Print and shaded views of the part. All mm, measured from the part's lowest x, y and z. A direction names the side the tool comes from. Give positions to 0.01 mm unless a question says otherwise; leave off trailing zeros. Write each loop counter-clockwise with the first axis right and the second up, starting at its lowest first coordinate (ties: lowest second). Pieces come first, ordered by that corner, then holes.
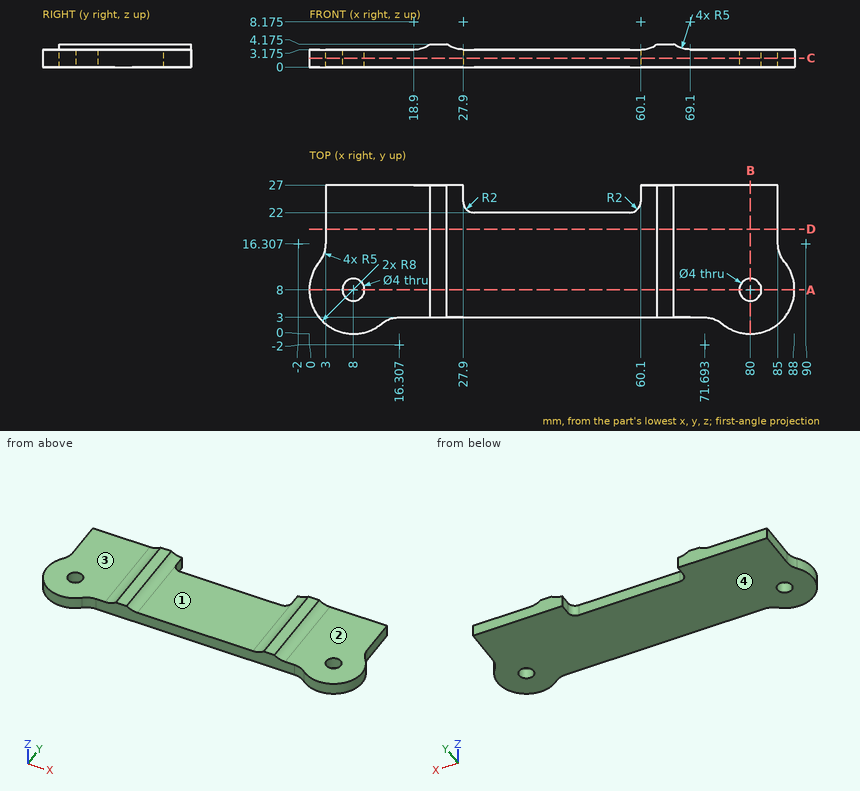
1. Drop flat-ended pins along their axis: pin 1 (9.5 mm diameter, centred on x = 79, y = 16.5, fed in from +Z) (3 decimals); pin 2 (1.6 mm diameter, centred on y = 20, z = 1, fed in from +X); pin 3 (3 mm diameter, centred on x = 80, y = 8, fed in from +Z); pin 4 (1.6 mm diameter, centred on y = 22.5, z = 1, fed in from -X). Give the stop position or say it passes through.
2. Saw through at B-B on x = 80. Give the cut face in (y, z) (1 decimal).
3. Mould opens along X. For the marked faces 1 and 2 say: pulls with the +X half, pulls with the -X half, needs draft (parallel to the pull), parting line crosses it, or undercut.
4. Saw through at D-D on y = 19. Give the cut face in (x, z) (1 decimal).
5. Drill centre lines: line 1 along Y through (x, z) = (80, 2.2); line 2 along Z through (x, y) = (74, 6.5) (1 decimal); line 3 along Y through (x, z) = (22, 1.8). Where is each one in solid material? Low to high.
6. Saw through at A-A on y = 8. Give the cut face in (x, z) (1 decimal).
7. 3-axis set-ups, long thin cutter, end or side, ignore diameter. For the marked faces 3 and 4: which of +Z, -Z, +X, -X, +Y, -Y reach the whole face in a straight line?
8. Saw through at C-C on z = 1.6. Give the cut face in (x, y).
Outcome:
1. pin 1: stops at z = 3.175
1. pin 2: stops at x = 85
1. pin 3: passes through
1. pin 4: stops at x = 3
2. outline: (0, 0) - (6, 0) - (6, 3.2) - (0, 3.2) - close; (10, 0) - (27, 0) - (27, 3.2) - (10, 3.2) - close
3. face 1: undercut
3. face 2: needs draft
4. outline: (3, 0) - (85, 0) - (85, 3.2) - (69.1, 3.2) arc R5 cw to (66.1, 4.2) - (63.1, 4.2) arc R5 cw to (60.1, 3.2) - (27.9, 3.2) arc R5 cw to (24.9, 4.2) - (21.9, 4.2) arc R5 cw to (18.9, 3.2) - (3, 3.2) - close
5. line 1: y = 0 to 6, 10 to 27
5. line 2: z = 0 to 3.2
5. line 3: y = 3 to 27
6. outline: (0, 0) - (6, 0) - (6, 3.2) - (0, 3.2) - close; (10, 0) - (78, 0) - (78, 3.2) - (69.1, 3.2) arc R5 cw to (66.1, 4.2) - (63.1, 4.2) arc R5 cw to (60.1, 3.2) - (27.9, 3.2) arc R5 cw to (24.9, 4.2) - (21.9, 4.2) arc R5 cw to (18.9, 3.2) - (10, 3.2) - close; (82, 0) - (88, 0) - (88, 3.2) - (82, 3.2) - close
7. face 3: +Z, -X, +Y, -Y
7. face 4: -Z, +X, -X, +Y, -Y
8. outline: (1.85, 13.11) arc R8 ccw to (13.11, 1.85) arc R5 cw to (16.31, 3) - (71.69, 3) arc R5 cw to (74.89, 1.85) arc R8 ccw to (86.15, 13.11) arc R5 cw to (85, 16.31) - (85, 27) - (60.1, 27) - (60.1, 24) arc R2 cw to (58.1, 22) - (29.9, 22) arc R2 cw to (27.9, 24) - (27.9, 27) - (3, 27) - (3, 16.31) arc R5 cw to start; hole circle Ø4 at (8, 8); hole circle Ø4 at (80, 8)
